from build123d import *

# Parameters (mm, degrees)
F0_R     = 12.7
F1_DEPTH = 1.524
F2_R     = 13.97
F3_DEPTH = 0.762
F4_W     = 5.08
F4_H     = 1.524
F6_W     = 5.08000508
F6_H     = 1.5265774739
F7_DEPTH = 0.508
F8_R     = 0.254


with BuildPart() as f1:
    # F0 (on Top) → F1 (new body)
    with BuildSketch(Plane.XY):
        Circle(F0_R)
    extrude(amount=-F1_DEPTH)

    # F2 (on Top) → F3 (join)
    with BuildSketch(Plane.XY):
        Circle(F2_R)
    extrude(amount=-F3_DEPTH)

    # F4 (on Front) → F5 (revolve, cut)
    with BuildSketch(Plane.XZ):
        Rectangle(F4_W, F4_H)
    revolve(axis=Axis((0, 0, 0.762), (-1, 0, 0)), mode=Mode.SUBTRACT)

    # F6 (on Top) → F7 (join)
    with BuildSketch(Plane.XY):
        Rectangle(F6_W, F6_H)
    extrude(amount=-F7_DEPTH)

    # F8
    f8_edges = [f1.edges().sort_by_distance(p)[0] for p in [
        (0, 0.763289, -0.508),
        (0, -0.763289, -0.508),
    ]]
    fillet(f8_edges, radius=F8_R)


solid = f1.part
Input: part model. Units: mm. Frame: model coordinates. A direction names the side the tool comes from. Coordinates: 2 decimals unless noted, no trailing zeros. Loops run counter-clockwise (first coordinate to the right, second up) from the corner with the lowest first, then second, coordinate; pieces in that order, holes last.
Q1. Set-up query: faces 4 (the face through (0.04, 0.02, -0.76)), 5 (the face through (0, 0, 0)). Return all of +Z, -Z, +X, -X, +Y, -Y with unobstructed straight access to the full face (end or side cutting, diameter ignored); none if empty.
Q2. Cut plane A-A (y = 0). Output: boundary loops of the cut face in (x, z), then the cut area to 3 significant figures.
Q3. Contact query for a flat-ended pin moving along its axis: pin 1 (6 mm diameter, centred on x = 9, y = -10, fed in from -Z). Output: stop coordinate, or through.
Q4. Draft query along X for faces 1 (the face through (0, 0, -0.508)), 2 (the face through (-2.75, -12.4, -1.14)), 3 (the face through (6.14, -11.32, -0.762)). Return one class per face: +X half, -X half, draft (parallel to the pull), parting line (faces both ways), or undercut.
Q5. Material intervals for line 1 (Y direction, x = -1.5, z = -0.3); line 2 (Z direction, x = -12.5, y = -2.75); line 3 (Y direction, x = 4.5, z = -0.4), sorted ascending.
Q6. Cut plane D-D (z = -1.2). Output: boundary loops of the cut face in (x, y).
Q7. Cut plane B-B (x = 0). Output: boundary loops of the cut face in (y, z), then the cut area to 3 significant figures.
Q8. Cut plane C-C (y = 5.5). Output: boundary loops of the cut face in (x, z).
Working result:
1. face 4: none
1. face 5: +Z, +X, -X, +Y, -Y
2. outline: (-13.97, -0.76) - (-12.7, -0.76) - (-12.7, -1.52) - (12.7, -1.52) - (12.7, -0.76) - (13.97, -0.76) - (13.97, 0) - (-13.97, 0) - close; hole (-2.54, -0.76) - (2.54, -0.76) - (2.54, -0.51) - (-2.54, -0.51) - close
2. area: 39.4 mm2
3. pin 1: stops at z = -1.52
4. face 1: undercut
4. face 2: parting line
4. face 3: draft
5. line 1: y = -13.89 to -1.09, -0.76 to 0.76, 1.09 to 13.89
5. line 2: z = -0.76 to 0
5. line 3: y = -13.23 to 13.23
6. outline: circle Ø25.4 at (0, 0)
7. outline: (-13.97, -0.76) - (-12.7, -0.76) - (-12.7, -1.52) - (12.7, -1.52) - (12.7, -0.76) - (13.97, -0.76) - (13.97, 0) - (1.32, 0) arc R1.52 cw to (-1.32, 0) - (-13.97, 0) - close; (-0.76, -0.25) arc R0.25 ccw to (-0.51, -0.51) - (0.51, -0.51) arc R0.25 ccw to (0.76, -0.25) - (0.76, 0) - (-0.76, 0) - close
7. area: 40.0 mm2
8. outline: (-12.84, -0.76) - (-11.45, -0.76) - (-11.45, -1.52) - (11.45, -1.52) - (11.45, -0.76) - (12.84, -0.76) - (12.84, 0) - (-12.84, 0) - close
